Autodesk Inventor part; units mm, degrees
ref_plane "YZ Plane" through (0, 0, 0) normal (1, 0, 0) x (0, 1, 0)
ref_plane "XZ Plane" through (0, 0, 0) normal (0, 1, 0) x (-1, 0, 0)
ref_plane "XY Plane" through (0, 0, 0) normal (0, 0, 1) x (1, 0, 0)
sketch "Sketch1" plane through (0, 0, 0) normal (0, 1, 0) x (-1, 0, 0)
  circle A0 centre (0, 0) radius 94
  dimension "d0" = 188
extrude "Extrusion1" add sketch "Sketch1" along normal blind 4
sketch "Sketch2" plane through (0, 4, 0) normal (0, 1, 0) x (1, 0, 0)
  circle A0 centre (0, 0) radius 87.5
  dimension "d3" = 175
hole "Hole1" at (0, 4, 0) direction (0, -1, 0) diameter 170 depth 2
sketch "Sketch3" plane through (0, 2, 0) normal (0, 1, 0) x (1, 0, 0)
  circle A0 centre (0, 0) radius 82
  dimension "d11" = 164
hole "Hole2" at (0, 2, 0) direction (0, -1, 0) diameter 165 end through all
sketch "Sketch4" plane through (0, 4, 0) normal (0, 1, 0) x (1, 0, 0)
  circle A0 centre (-90, 0) radius 1.65
  point P0 (0, 0)
  dimension "d19" = 3.3
  dimension "d20" = 90
sketch "Sketch5" plane through (0, 4, 0) normal (0, 1, 0) x (1, 0, 0)
  circle A0 centre (-63.6396, 63.6396) radius 1.65
  point P0 (0, 0)
  dimension "d28" = 3.3
  dimension "d29" = 90
  dimension "d33" = 63.6396
sketch "Sketch6" plane through (0, 4, 0) normal (0, 1, 0) x (1, 0, 0)
  circle A0 centre (0, 90) radius 1.65
  point P0 (0, 0)
  dimension "d34" = 3.3
  dimension "d35" = 90
sketch "Sketch7" plane through (0, 4, 0) normal (0, 1, 0) x (1, 0, 0)
  circle A0 centre (63.6396, 63.6396) radius 1.65
  point P0 (0, 0)
  dimension "d36" = 3.3
  dimension "d37" = 90
  dimension "d38" = 63.6396
  dimension "d121" = 63.6396
sketch "Sketch8" plane through (0, 4, 0) normal (0, 1, 0) x (1, 0, 0)
  circle A0 centre (90, 0) radius 1.65
  point P0 (0, 0)
  dimension "d39" = 3.3
  dimension "d40" = 90
sketch "Sketch9" plane through (0, 4, 0) normal (0, 1, 0) x (1, 0, 0)
  circle A0 centre (63.6396, -63.6396) radius 2.15
  point P0 (0, 0)
  dimension "d41" = 4.3
  dimension "d42" = 90
  dimension "d43" = 63.6396
  dimension "d122" = 63.6396
sketch "Sketch10" plane through (0, 4, 0) normal (0, 1, 0) x (1, 0, 0)
  circle A0 centre (0, -90) radius 1.65
  point P0 (0, 0)
  dimension "d44" = 3.3
  dimension "d45" = 90
sketch "Sketch11" plane through (0, 4, 0) normal (0, 1, 0) x (1, 0, 0)
  circle A0 centre (-63.6396, -63.6396) radius 1.65
  point P0 (0, 0)
  dimension "d46" = 3.3
  dimension "d47" = 90
  dimension "d48" = 63.6396
  dimension "d123" = 63.6396
hole "Hole4" at (-90, 4, 0) direction (0, -1, 0) diameter 3.3 end through all
hole "Hole5" at (-63.6396, 4, -63.6396) direction (0, -1, 0) diameter 3.3 end through all
hole "Hole6" at (0, 4, -90) direction (0, -1, 0) diameter 3.3 end through all
hole "Hole7" at (63.6396, 4, -63.6396) direction (0, -1, 0) diameter 3.3 end through all
hole "Hole8" at (90, 4, 0) direction (0, -1, 0) diameter 3.3 end through all
hole "Hole9" at (63.6396, 4, 63.6396) direction (0, -1, 0) diameter 3.3 end through all
hole "Hole10" at (0, 4, 90) direction (0, -1, 0) diameter 3.3 end through all
hole "Hole11" at (-63.6396, 4, 63.6396) direction (0, -1, 0) diameter 3.3 end through all
thread "Thread9"
thread "Thread10"
thread "Thread11"
thread "Thread12"
thread "Thread13"
thread "Thread14"
thread "Thread15"
thread "Thread16"
thread "Thread17"
properties part number "Shield Support Ring"
Can you work these out from the model? Positions are in its coordinate system, mm. A direction names the side the tool comes from. Give positions to 0.01 mm unless a question says otherwise; leave off trailing zeros. Loops run counter-clockwise (first coordinate to the right, second up) from the corner with the lowest first, then second, coordinate; pieces in that order, holes last. Notation, with made-up numbers: (44, 64) - (78, 64) arc R10 ccw to (78, 71) - close; hole circle Ø4 at (5, 55). An arc over 180 degrees is marked (long way). Return JSON: item names as keys, results as strings.
1. If I drill on line 1 (Z direction, x = 0, y = 0.5); line 2 (Y direction, x = 22, z = -80); line 3 (X direction, y = 2.15, z = 14), over which ranges is the centre line in solid material (lowest first)?
Output values:
{"line 1": "z = -94 to -91.65, -88.35 to -82.5, 82.5 to 88.35, 91.65 to 94", "line 2": "y = 0 to 2", "line 3": "x = -92.95 to -83.84, 83.84 to 92.95"}
2. I'm going to push flat-ended pins straight in: pin 1 Ø2 at (y, z) = (1.5, 42) entering from +X; pin 2 Ø1 at (y, z) = (2, -67) entering from -X. Where does each tip first touch, or does it pass through?
Output values:
{"pin 1": "stops at x = 84.59", "pin 2": "stops at x = -66.44"}
3. I want a section at B-B on x = -13. Please give me the cut outline in (y, z).
Output values:
{"outline": "(0, -93.1) - (4, -93.1) - (4, -84) - (2, -84) - (2, -81.47) - (0, -81.47) - close; (0, 81.47) - (2, 81.47) - (2, 84) - (4, 84) - (4, 93.1) - (0, 93.1) - close"}
4. I want a section at C-C on y = 3. Give the number of separate pieces and of enclosed holes in the cut face, and give its area (3 significant figures).
Output values:
{"separate pieces": "1", "enclosed holes": "9", "area": "4,990 mm²"}
5. We'd pull the mould along X, two halves only. Please class faces 3 (the face through (51.721, 2.986, -67.453)), 4 (the face through (84, 4, 14)), 5 (the face through (80.54, 0.99, -17.88)), 6 (the face through (-89.659, 1.972, -28.235)): +X half, -X half, draft (parallel to the pull), parting line (faces both ways), or undercut.
Output values:
{"face 3": "undercut", "face 4": "draft", "face 5": "undercut", "face 6": "parting line"}
6. I want a section at A-A on z = -56.5. Please give me the cut outline in (x, y).
Output values:
{"outline": "(-75.12, 0) - (-60.12, 0) - (-60.12, 2) - (-63.5, 2) - (-63.5, 4) - (-75.12, 4) - close; (60.12, 0) - (75.12, 0) - (75.12, 4) - (63.5, 4) - (63.5, 2) - (60.12, 2) - close"}
7. For faces 1 (the face through (-55, 0, -62)), 2 (the face through (-70, 2, -44)), which set-ups out of +Z, -Z, +X, -X, +Y, -Y let a thin tool reach every point of the face, with its end or its side?
Output values:
{"face 1": "+Z, -Z, +X, -X, -Y", "face 2": "+Y"}
